Here's how the part is built. I have some questions about the finished solid (model axes, mm). A direction names the side the tool comes from. Coordinates: 2 decimals unless noted, no trailing zeros. Order: outer loops, then holes, each group sorted by start corner. A loop starts at its lowest first (then second) coordinate and runs counter-clockwise, first axis right, second up. Notation, with made-up numbers: M 40.5,81.5 L 91.5,81.5 A17 cw 91.5,103.5 Z; hole C 12,10.5 d10. An arc over 180 degrees is marked long. One line per question, with ' | ' between items. Start each with the question number.
```python
from build123d import *

# Parameters (mm, degrees)
SKETCH1_W                   = 100
SKETCH1_H                   = 10
BOSS_EXTRUDE1_DEPTH         = 15
SKETCH2_R                   = 7.5
BOSS_EXTRUDE2_DEPTH         = 20
SKETCH3_W                   = 18.5
SKETCH3_H                   = 18.5
BOSS_EXTRUDE3_DEPTH         = 20
CHAMFER1_SIZE               = 3
CHAMFER2_SIZE               = 5
SKETCH4_W                   = 11.2
SKETCH4_H                   = 5.65
CUT_EXTRUDE1_DEPTH          = 116.616824035
F_1_4_CLEARANCE_HOLE1_D     = 7.14248
F_1_4_CLEARANCE_HOLE1_DEPTH = 25
F_1_4_CLEARANCE_HOLE1_TIP   = 2.145817477
SKETCH8_W                   = 15
SKETCH8_H                   = 15
BOSS_EXTRUDE4_DEPTH         = 5
SKETCH9_R                   = 2.65
CUT_EXTRUDE2_DEPTH          = 25
F_4_CLEARANCE_HOLE1_D       = 3.4544
F_4_CLEARANCE_HOLE1_DEPTH   = 10
F_4_CLEARANCE_HOLE1_TIP     = 1.037806461
SKETCH13_W                  = 6.6
SKETCH13_H                  = 2.79
CUT_EXTRUDE3_DEPTH          = 7.7559
SKETCH14_W                  = 15
SKETCH14_H                  = 15
BOSS_EXTRUDE5_DEPTH         = 3
SKETCH15_W                  = 2.5
SKETCH15_H                  = 15
CUT_EXTRUDE4_DEPTH          = 42.5
SKETCH16_W                  = 2.5
SKETCH16_H                  = 15
CUT_EXTRUDE5_DEPTH          = 42.5


with BuildPart() as part:
    # Sketch1 → Boss-Extrude1 (new body)
    with BuildSketch(Plane(origin=(0, 0, 0), x_dir=(1, 0, 0), z_dir=(0, 1, 0))):
        with Locations((50, 5)):
            Rectangle(SKETCH1_W, SKETCH1_H)
    extrude(amount=BOSS_EXTRUDE1_DEPTH)

    # Sketch2 → Boss-Extrude2 (add)
    with BuildSketch(Plane(origin=(0, 15, 0), x_dir=(1, 0, 0), z_dir=(0, 1, 0))):
        with Locations(Location((50, 5, 0), (0, 0, 41.810314896))):
            Circle(SKETCH2_R)
    extrude(amount=BOSS_EXTRUDE2_DEPTH)

    # Sketch3 → Boss-Extrude3 (add)
    with BuildSketch(Plane(origin=(0, 35, 0), x_dir=(1, 0, 0), z_dir=(0, 1, 0))):
        with Locations((50, 5)):
            Rectangle(SKETCH3_W, SKETCH3_H)
    extrude(amount=BOSS_EXTRUDE3_DEPTH)

    # Chamfer1
    chamfer1_edges = [part.edges().sort_by_distance(p)[0] for p in [
        (40.75, 55, -5),
        (50, 55, 4.25),
        (59.25, 55, -5),
        (50, 55, -14.25),
    ]]
    chamfer(chamfer1_edges, length=CHAMFER1_SIZE)

    # Chamfer2
    # the kernel refuses this chamfer: 5 mm, written as the material it takes off along each edge
    with BuildSketch(Plane(origin=(27.89158506, 35, -14.25), x_dir=(0, 0.9996219169112968, -0.027495876610586317), z_dir=(1, 0, 0))) as chamfer2_piece_1_section:
        Polygon((CHAMFER2_SIZE * 0.999621916911, CHAMFER2_SIZE * 0.0274958766106), (-CHAMFER2_SIZE * 0.0274958766106, CHAMFER2_SIZE * 0.999621916911), (0, 0), align=None)
    chamfer2_piece_1 = extrude(amount=44.21682988, mode=Mode.PRIVATE)
    chamfer2_piece_1 = chamfer2_piece_1 - Plane(origin=(50, 36.70985324, -5), x_dir=(0.7453559924973537, 0, -0.6666666666695469), z_dir=(0, -1, 0)) * Cylinder(7.5, 109, mode=Mode.PRIVATE)
    with BuildSketch(Plane(origin=(40.75, 35, 17.10841494), x_dir=(-0.027495876610586317, 0.9996219169112968, 0), z_dir=(0, 0, -1))) as chamfer2_piece_2_section:
        Polygon((CHAMFER2_SIZE * 0.999621916911, CHAMFER2_SIZE * 0.0274958766106), (-CHAMFER2_SIZE * 0.0274958766106, CHAMFER2_SIZE * 0.999621916911), (0, 0), align=None)
    chamfer2_piece_2 = extrude(amount=44.21682988, mode=Mode.PRIVATE)
    chamfer2_piece_2 = chamfer2_piece_2 - Plane(origin=(50, 36.709853278, -5), x_dir=(0.7453559924973537, 0, -0.6666666666695469), z_dir=(0, -1, 0)) * Cylinder(7.5, 109, mode=Mode.PRIVATE)
    with BuildSketch(Plane(origin=(59.25, 35, -27.10841494), x_dir=(-0.9996219169112968, -0.027495876610586317, 0), z_dir=(0, 0, 1))) as chamfer2_piece_3_section:
        Polygon((CHAMFER2_SIZE * 0.999621916911, -CHAMFER2_SIZE * 0.0274958766106), (-CHAMFER2_SIZE * 0.0274958766106, -CHAMFER2_SIZE * 0.999621916911), (0, 0), align=None)
    chamfer2_piece_3 = extrude(amount=44.21682988, mode=Mode.PRIVATE)
    chamfer2_piece_3 = chamfer2_piece_3 - Plane(origin=(50, 36.709853248, -5), x_dir=(0.7453559924973537, 0, -0.6666666666695469), z_dir=(0, -1, 0)) * Cylinder(7.5, 109, mode=Mode.PRIVATE)
    with BuildSketch(Plane(origin=(72.10841494, 35, 4.25), x_dir=(0, -0.027495876610586317, -0.9996219169112968), z_dir=(-1, 0, 0))) as chamfer2_piece_4_section:
        Polygon((CHAMFER2_SIZE * 0.999621916911, -CHAMFER2_SIZE * 0.0274958766106), (-CHAMFER2_SIZE * 0.0274958766106, -CHAMFER2_SIZE * 0.999621916911), (0, 0), align=None)
    chamfer2_piece_4 = extrude(amount=44.21682988, mode=Mode.PRIVATE)
    chamfer2_piece_4 = chamfer2_piece_4 - Plane(origin=(50, 36.709853226, -5), x_dir=(0.7453559924973537, 0, -0.6666666666695469), z_dir=(0, -1, 0)) * Cylinder(7.5, 109, mode=Mode.PRIVATE)
    add([chamfer2_piece_1, chamfer2_piece_2, chamfer2_piece_3, chamfer2_piece_4], mode=Mode.SUBTRACT)

    # Sketch4 → Cut-Extrude1 (cut, through all)
    with BuildSketch(Plane.XY.offset(4.25)):
        with Locations((50, 46)):
            Rectangle(SKETCH4_W, SKETCH4_H)
    extrude(amount=-CUT_EXTRUDE1_DEPTH, mode=Mode.SUBTRACT)

    # 1/4 Clearance Hole1
    with Locations(Plane(origin=(0, 55, 0), x_dir=(1, 0, 0), z_dir=(0, 1, 0))):
        with Locations((50, 5)):
            Hole(F_1_4_CLEARANCE_HOLE1_D / 2, depth=F_1_4_CLEARANCE_HOLE1_DEPTH)
            with Locations((0, 0, -(F_1_4_CLEARANCE_HOLE1_DEPTH + F_1_4_CLEARANCE_HOLE1_TIP / 2))):  # 118° drill point
                Cone(0, F_1_4_CLEARANCE_HOLE1_D / 2, F_1_4_CLEARANCE_HOLE1_TIP, mode=Mode.SUBTRACT)

    # Sketch8 → Boss-Extrude4 (add)
    with BuildSketch(Plane.XY):
        with Locations((50, 7.5)):
            Rectangle(SKETCH8_W, SKETCH8_H)
    extrude(amount=BOSS_EXTRUDE4_DEPTH)

    # Sketch9 → Cut-Extrude2 (cut)
    with BuildSketch(Plane.XZ):
        with Locations(Location((50, -5, 0), (0, 0, 270))):
            Circle(SKETCH9_R)
    extrude(amount=-CUT_EXTRUDE2_DEPTH, mode=Mode.SUBTRACT)

    # #4 Clearance Hole1
    with Locations(Plane.XY.offset(5)):
        with Locations((50, 5)):
            Hole(F_4_CLEARANCE_HOLE1_D / 2, depth=F_4_CLEARANCE_HOLE1_DEPTH)
            with Locations((0, 0, -(F_4_CLEARANCE_HOLE1_DEPTH + F_4_CLEARANCE_HOLE1_TIP / 2))):  # 118° drill point
                Cone(0, F_4_CLEARANCE_HOLE1_D / 2, F_4_CLEARANCE_HOLE1_TIP, mode=Mode.SUBTRACT)

    # Sketch13 → Cut-Extrude3 (cut)
    with BuildSketch(Plane.XZ):
        with Locations((50, 1.105)):
            Rectangle(SKETCH13_W, SKETCH13_H)
    extrude(amount=-CUT_EXTRUDE3_DEPTH, mode=Mode.SUBTRACT)

    # Sketch14 → Boss-Extrude5 (add)
    with BuildSketch(Plane(origin=(0, 0, -10), x_dir=(-1, 0, 0), z_dir=(0, 0, -1))):
        with Locations((-50, 7.5)):
            Rectangle(SKETCH14_W, SKETCH14_H)
    extrude(amount=BOSS_EXTRUDE5_DEPTH)

    # Sketch15 → Cut-Extrude4 (cut)
    with BuildSketch(Plane(origin=(100, 0, 0), x_dir=(0, 0, -1), z_dir=(1, 0, 0))):
        with Locations((1.25, 7.5)):
            Rectangle(SKETCH15_W, SKETCH15_H)
        with Locations((8.75, 7.5)):
            Rectangle(SKETCH15_W, SKETCH15_H)
    extrude(amount=-CUT_EXTRUDE4_DEPTH, mode=Mode.SUBTRACT)

    # Sketch16 → Cut-Extrude5 (cut)
    with BuildSketch(Plane.ZY):
        with Locations((-8.75, 7.5)):
            Rectangle(SKETCH16_W, SKETCH16_H)
        with Locations((-1.25, 7.5)):
            Rectangle(SKETCH16_W, SKETCH16_H)
    extrude(amount=-CUT_EXTRUDE5_DEPTH, mode=Mode.SUBTRACT)


solid = part.part
```
1. Will these pins go through, and if not, where does the flat tip stop? pin 1 (1.7 mm diameter, centred on y = 45.5, z = -9.5, fed in from +X); pin 2 (16.5 mm diameter, centred on x = 48.5, y = 9, fed in from -Z); pin 3 (2 mm diameter, centred on y = 3, z = 1, fed in from +X); pin 4 (8 mm diameter, centred on x = 66.5, y = 39.5, fed in from +Z).
2. I need wall thicknesses on line 1 (X direction, y = 5, z = -1.2); line 2 (Y direction, x = 54, z = -4.5) (3 decimals); line 3 (X direction, y = 10, z = -4.75). Which ranges of each line are inside material? Lowest first, please.
3. Imagine slicing it at C-C (y = 26.5). List the corners of the cut face in (x, z) for me, then the cut area to 3 significant figures.
4. We'd pull the mould along Z, two halves only. Please class faces 4 (the face through (44.4, 46, -5)), 5 (the face through (50, 7.756, 1)), 6 (the face through (79, 7, -7.5)): released by +Z, released by -Z, zero draft, split by the parting line, or undercut.
5. Imagine slicing it at A-A (y = 5). List the corners of the cut face in (x, z) for me, then the cut area to 3 significant figures.
6. Imagine slicing it at B-B (x = 15). List the corners of the cut face in (y, z) for me, then the cut area to 3 significant figures.
7. Which directions (+Z, -Z, +X, -X, +Y, -Y) give clear straight access to the entire face, cutting with the end or side of a thin tool? Please do faces 1 (the face through (57.5, 7, -10)), 2 (the face through (48.405, 4.338, 3.732)), 3 (the face through (50.796, 12.325, -7.528)).
Entries:
1) pin 1: x = 59.25 | pin 2: z = -13 | pin 3: x = 57.5 | pin 4: through
2) line 1: 42.5 to 48.27, 51.73 to 57.5 | line 2: 0 to 43.175, 48.825 to 55 | line 3: 0 to 47.36, 52.64 to 100
3) outline: C 50,-5 d15 | area: 177 mm²
4) face 4: zero draft | face 5: undercut | face 6: released by -Z
5) outline: M 0,-7.5 L 42.5,-7.5 L 42.5,-13 L 57.5,-13 L 57.5,-7.5 L 100,-7.5 L 100,-2.5 L 57.5,-2.5 L 57.5,5 L 51.73,5 L 51.73,2.5 L 53.3,2.5 L 53.3,-0.29 L 51.73,-0.29 L 51.73,-2.99 A2.65 cw long 48.27,-2.99 L 48.27,-0.29 L 46.7,-0.29 L 46.7,2.5 L 48.27,2.5 L 48.27,5 L 42.5,5 L 42.5,-2.5 L 0,-2.5 Z | area: 638 mm²
6) outline: M 0,-7.5 L 15,-7.5 L 15,-2.5 L 0,-2.5 Z | area: 75.0 mm²
7) face 1: -Z, +X, -Y | face 2: +Z | face 3: -Y
